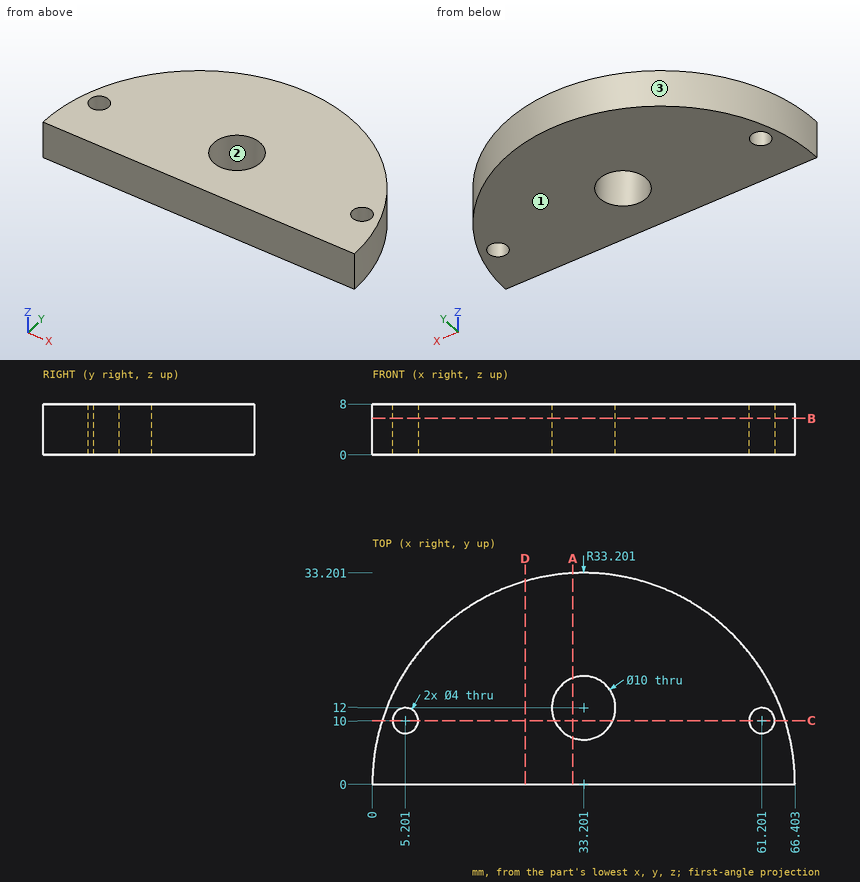
The figure shows three views and two pictorial views of one solid part (mm, origin at its lowest corner). Answer the questions. Give positions to 0.01 mm unless a question says otherwise; leave off trailing zeros. Loops run counter-clockwise (first coordinate to the right, second up) from the corner with the lowest first, then second, coordinate; pieces in that order, holes last. Notation, with made-up numbers: (-34, 18) - (-28, 18) arc R11 cw to (-28, 38) - close; hole circle Ø6 at (59.5, 66.25). An arc over 180 degrees is marked (long way). Answer in a Markdown table with one row per item.
(1) Section D-D (x = 24) is taken. Give the vertices of the cut face in (y, z), and give its area (3 significant figures).
Results list:
| item | result |
|---|---|
| outline | (0, 0) - (31.9, 0) - (31.9, 8) - (0, 8) - close |
| area | 255 mm² |
(2) For a pull along X with two mould halves and no side action, classify the marked faces 1, 2 and 3 as pulls with the +X half, pulls with the -X half, needs draft (parallel to the pull), parting line crosses it, or undercut.
Results list:
| item | result |
|---|---|
| face 1 | needs draft |
| face 2 | undercut |
| face 3 | parting line crosses it |
(3) Consider L1, parallel to Y at x = 33, z = 4.5; L2, parallel to Y at x = 29.5, z = 1 (1 decimal); L3, parallel to Y at x = 42.5, z = 3.75. Determine where each line is inside the solid, lowest interval first. Write a range as [from, to].
Results list:
| item | result |
|---|---|
| L1 | y = [0, 7], [17, 33.2] |
| L2 | y = [0, 8.6], [15.4, 33] |
| L3 | y = [0, 31.87] |
(4) Section B-B (z = 5.75) is taken. Give the vertices of the cut face in (x, y).
Results list:
| item | result |
|---|---|
| outline | (0, 0) - (66.4, 0) arc R33.2 ccw to start; hole circle Ø4 at (5.2, 10); hole circle Ø10 at (33.2, 12); hole circle Ø4 at (61.2, 10) |
(5) Section C-C (y = 10) is taken. Give the vertices of the cut face in (x, z).
Results list:
| item | result |
|---|---|
| outline | (1.54, 0) - (3.2, 0) - (3.2, 8) - (1.54, 8) - close; (7.2, 0) - (28.62, 0) - (28.62, 8) - (7.2, 8) - close; (37.78, 0) - (59.2, 0) - (59.2, 8) - (37.78, 8) - close; (63.2, 0) - (64.86, 0) - (64.86, 8) - (63.2, 8) - close |
(6) Section A-A (x = 31.5) is taken. Give the vertices of the cut face in (y, z).
Results list:
| item | result |
|---|---|
| outline | (0, 0) - (7.3, 0) - (7.3, 8) - (0, 8) - close; (16.7, 0) - (33.16, 0) - (33.16, 8) - (16.7, 8) - close |
(7) Flat-ended cylindrical pins translate along their axes: pin 1 Ø5 at (x, y) = (48, 24.5) entering from -Z; pin 2 Ø1.5 at (y, z) = (18.5, 5.5) entering from -X; pin 3 Ø4 at (x, z) = (57.5, 5) entering from +Y; pin 4 Ø2 at (y, z) = (22.5, 6) entering from +X. Find the tip coordinate at first contact, or state that the pin passes through.
Results list:
| item | result |
|---|---|
| pin 1 | stops at z = 0 |
| pin 2 | stops at x = 5.14 |
| pin 3 | stops at y = 24.6 |
| pin 4 | stops at x = 58.5 |
